Part model, mm, in its own coordinate system. Give positions to 0.01 mm unless a question says otherwise; leave off trailing zeros. Loops run counter-clockwise (first coordinate to the right, second up) from the corner with the lowest first, then second, coordinate; pieces in that order, holes last. Notation, with made-up numbers: (-21, 19) -> (0, 19) arc R37 ccw to (0, 58) -> close; hole circle Ø7 at (25, 59.25). An arc over 180 degrees is marked (long way). One line per question, with ' | ' between items.
```python
from build123d import *

# Parameters (mm, degrees)
F0_W     = 45.72
F0_H     = 143.256
F1_DEPTH = 4.064
F2_SIZE2 = 0.762
F2_SIZE  = 0.762
F4_D     = 20.32


with BuildPart() as f1:
    # F0 (on Front) → F1 (new body)
    with BuildSketch(Plane.XZ):
        Rectangle(F0_W, F0_H)
    extrude(amount=F1_DEPTH)

    # F2
    f2_edges = [f1.edges().sort_by_distance(p)[0] for p in [
        (22.86, -2.032, 71.628),
        (-22.86, -2.032, 71.628),
        (-22.86, -2.032, -71.628),
        (22.86, -2.032, -71.628),
    ]]
    chamfer(f2_edges, length=F2_SIZE, length2=F2_SIZE2)

    # F4 (through all)
    with Locations(Plane.XZ.offset(4.064)):
        with Locations((0, 55.372)):
            Hole(F4_D / 2)


solid = f1.part
```
1) Saw through at A-A (x = 0). Give the cut face in (y, z), and give its area (3 significant figures).
Found:
outline: (-4.06, -71.63) -> (0, -71.63) -> (0, 45.21) -> (-4.06, 45.21) -> close; (-4.06, 65.53) -> (0, 65.53) -> (0, 71.63) -> (-4.06, 71.63) -> close | area: 500 mm2
2) Saw through at B-B (y = -2.9). Give the cut face in (x, z), and give its area (3 significant figures).
Found:
outline: (-22.86, -70.87) -> (-22.1, -71.63) -> (22.1, -71.63) -> (22.86, -70.87) -> (22.86, 70.87) -> (22.1, 71.63) -> (-22.1, 71.63) -> (-22.86, 70.87) -> close; hole circle Ø20.32 at (0, 55.37) | area: 6,220 mm2
3) Drill centre lines: line 1 (Z direction, x = 0, y = -2); line 2 (X direction, y = -0.6, z = 55.5); line 3 (X direction, y = -3.1, z = 54.5). Where is each one in solid material? Low to high.
Found:
line 1: -71.63 to 45.21, 65.53 to 71.63 | line 2: -22.86 to -10.16, 10.16 to 22.86 | line 3: -22.86 to -10.12, 10.12 to 22.86
4) Pull direction X, two halves, no side cores. Call faces 1 (the cylindrical face through (2.202, -2.004, 45.454)), 2 (the flat face through (0, -2, 71.628)), 3 (the flat face through (-22.86, -2, -1)): pulls with the +X half, pulls with the -X half, needs draft (parallel to the pull), parting line crosses it, or undercut.
Found:
face 1: undercut | face 2: needs draft | face 3: pulls with the -X half
5) Saw through at C-C (z = 63). Give the cut face in (x, y), and give its area (3 significant figures).
Found:
outline: (-22.86, -4.06) -> (-6.71, -4.06) -> (-6.71, 0) -> (-22.86, 0) -> close; (6.71, -4.06) -> (22.86, -4.06) -> (22.86, 0) -> (6.71, 0) -> close | area: 131 mm2
